Geometry: final body of the model. Coordinates: model frame, mm. Face numbers are marked on the shaded views. Coordinates: 2 decimals unless noted, no trailing zeros. Write each loop counter-clockwise with the first axis right and the second up, starting at its lowest first coordinate (ties: lowest second). Pieces come first, ordered by that corner, then holes. Notation, with made-up numbers: (29.25, -20) - (61.25, -20) arc R16 cw to (61.25, -14) - close; hole circle Ø6 at (63, 84.25). An arc over 180 degrees is marked (long way). Answer as a JSON object with one key per item and string values. Group by question number.
Item 1: Section C-C on y = 11.5. Return loops of the section in (x, z).
Item 2: Line query: line 1 along Y through (x, z) = (0.5, 17); line 2 along Y through (x, z) = (-5.5, -9.5); line 3 along X through (y, z) = (9, -12). Output: solid intervals per line, ascending. Write a range as from..to.
Item 3: Section B-B on y = 0. Return loops of the section in (x, z), and give its area (3 significant figures).
Item 4: First-contact query: pin 1 Ø12 at (x, z) = (-7, 12.5) entering from -Y; pin 2 Ø6 at (x, z) = (5, -13) entering from +Y; pin 3 Ø12 at (x, y) = (7, 6) entering from +Z; pin 4 Ø5 at (y, z) = (-13.5, -14) entering from -X. Flat tips, straight axial feed; report the tip coordinate or a pass-through.
Item 5: Mould query, pull axis Y, two halves, no side actions, for the marked faces 1 and 2. Classes: pulls with the +Y half, pulls with the -Y half, needs draft (parallel to the pull), parting line crosses it, or undercut.
Item 6: Section A-A on x = 0. Return loops of the section in (y, z).
Item 7: Section D-D on z = 0. Return loops of the section in (x, y), and give its area (3 significant figures).
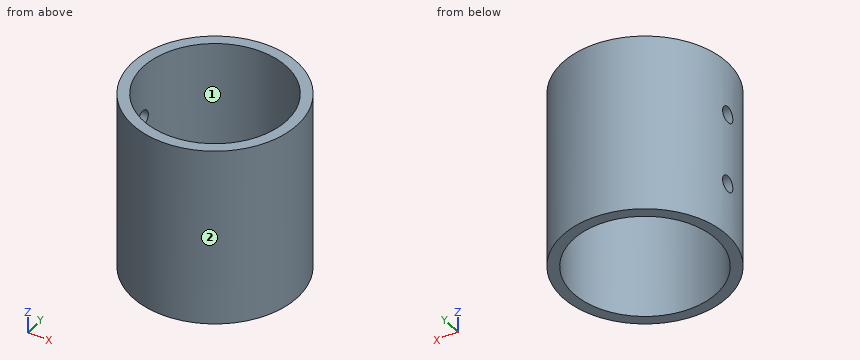
Autodesk Inventor part; units mm, degrees
ref_plane "YZ Plane" through (0, 0, 0) normal (1, 0, 0) x (0, 1, 0)
ref_plane "XZ Plane" through (0, 0, 0) normal (0, 1, 0) x (-1, 0, 0)
ref_plane "XY Plane" through (0, 0, 0) normal (0, 0, 1) x (1, 0, 0)
sketch "Sketch1" plane through (0, 0, 0) normal (0, 0, 1) x (1, 0, 0)
  circle A0 centre (0, 0) radius 20
  circle A1 centre (0, 0) radius 23
  dimension "d0" = 40
  dimension "d1" = 46
extrude "Extrusion1" add sketch "Sketch1" along normal mid plane 50
sketch "Sketch2" plane through (0, 0, 0) normal (1, 0, 0) x (0, 1, 0)
  line L0 (0, 105) -> (0, -105)
  line L1 (-105, 0) -> (105, 0)
  line L2 (23, 25) -> (-23, 25)
  line L3 (-23, -25) -> (23, -25)
  point P0 (0, 0)
  point P1 (0, 10)
  point P2 (0, -10)
  point P3 (0, -25)
  dimension "d21" = 20
  dimension "d22" = 15
hole "Hole1" at (0, 0, 10) at (0, 0, -10) direction (-1, 0, 0) diameter 4.5 end through all
sketch "Sketch3" plane through (0, 0, 0) normal (1, 0, 0) x (0, 1, 0)
  line L0 (23, -25) -> (7, -25)
  line L1 (7, -25) -> (7, 25)
  line L2 (7, 25) -> (23, 25)
  line L3 (23, 25) -> (23, -25)
  line L4 (23, 25) -> (-23, 25)
  line L5 (-23, -25) -> (23, -25)
  line L6 (0, 195.3) -> (0, -195.3)
  point P0 (0, 0)
  dimension "d13" = 0
  dimension "d14" = 0
  dimension "d15" = 7
extrude "Extrusion2" [suppressed]
properties part number "Top_Separator Pipe" material "PVC-Piping"
Checks:
{
 "1": {"outline": "(-19.92, -25) - (-16.36, -25) - (-16.36, 25) - (-19.92, 25) - close; (16.36, -25) - (19.92, -25) - (19.92, 25) - (16.36, 25) - close"},
 "2": {"line 1": "-22.99..-19.99, 19.99..22.99", "line 2": "-22.33..-19.23, 19.23..22.33", "line 3": "-21.17..-17.86, 17.86..21.17"},
 "3": {"outline": "(-23, -25) - (-20, -25) - (-20, -12.25) - (-23, -12.25) - close; (-23, -7.75) - (-20, -7.75) - (-20, 7.75) - (-23, 7.75) - close; (-23, 12.25) - (-20, 12.25) - (-20, 25) - (-23, 25) - close; (20, -25) - (23, -25) - (23, 25) - (20, 25) - close", "area": "273 mm^2"},
 "4": {"pin 1": "y = -22.98", "pin 2": "y = 22.91", "pin 3": "through", "pin 4": "x = -20.2"},
 "5": {"face 1": "undercut", "face 2": "parting line crosses it"},
 "6": {"outline": "(-23, -25) - (-20, -25) - (-20, 25) - (-23, 25) - close; (20, -25) - (23, -25) - (23, 25) - (20, 25) - close"},
 "7": {"outline": "circle Ø46 at (0, 0); hole circle Ø40 at (0, 0)", "area": "405 mm^2"}
}
